Input: part model. Units: mm. Frame: model coordinates. A direction names the side the tool comes from. Round coordinates to 2 decimals unless told otherwise and drop trailing zeros. Order: outer loops, then holes, each group sorted by start corner. A loop starts at its lowest first (then second) coordinate and runs counter-clockwise, first axis right, second up. Notation, with made-up numbers: (38.5, 56) - (58.5, 56) arc R23 cw to (58.5, 93) - close; hole circle Ø2 at (1.5, 87.5). An arc over 180 degrees is marked (long way). One line per item, written item: value. Start each with the question number.
from build123d import *

# Parameters (mm, degrees)
F0_W     = 132.842
F0_H     = 119.38
F1_DEPTH = 88.392
F2_R     = 40.132
F3_DEPTH = 120.396
F4_R     = 9.525
F5_DEPTH = 79.502


with BuildPart() as f1:
    # F0 (on Front) → F1 (new body)
    with BuildSketch(Plane.XZ):
        with Locations((-0.909254, 5.516134)):
            Rectangle(F0_W, F0_H)
    extrude(amount=-F1_DEPTH)

    # F2 (on face) → F3 (join)
    with BuildSketch(Plane.XY.offset(65.206134)):
        with Locations((40.111746, 37.592)):
            Circle(F2_R)
    extrude(amount=F3_DEPTH)

    # F4 (on face) → F5 (join)
    with BuildSketch(Plane.XZ):
        with Locations((-12.720254, 1.706134)):
            Circle(F4_R)
    extrude(amount=F5_DEPTH)


solid = f1.part
1. Pin query (flat end, axial travel): pin 1 (1.5 mm diameter, centred on y = 70, z = 31, fed in from +X); pin 2 (6 mm diameter, centred on x = 15, z = 134, fed in from -Y); pin 3 (3 mm diameter, centred on x = 38, z = 66.5, fed in from -Y). Return the tip coordinate at first contact, or that it passes through.
2. Section B-B (x = -32.5). Return the cut outline in (y, z).
3. Section D-D (z = 134). Return the cut outline in (x, y).
4. Line query: line 1 (Y direction, x = -20, z = -43.5); line 2 (Z direction, x = -13.5, y = 39); line 3 (X direction, y = 61, z = -3.5). Output: solid intervals per line, ascending. Write a range as from..to.
5. Section C-C (y = -52). Return the cut outline in (x, z) (3 decimals).
6. Set-up query: faces 1 (the face through (62, 2, 65.206)), 2 (the face through (65.512, 44, 5)), 3 (the face through (-3.635, -39.194, 4.567)). Return all of +Z, -Z, +X, -X, +Y, -Y with unobstructed straight access to the full face (end or side cutting, diameter ignored); none if empty.
7. Section A-A (z = 62.5). Return the cut outline in (x, y).
Solved:
1. pin 1: stops at x = 65.51
1. pin 2: stops at y = 4.1
1. pin 3: stops at y = -2.54
2. outline: (0, -54.17) - (88.39, -54.17) - (88.39, 65.21) - (0, 65.21) - close
3. outline: circle Ø80.26 at (40.11, 37.59)
4. line 1: y = 0..88.39
4. line 2: z = -54.17..65.21
4. line 3: x = -67.33..65.51
5. outline: circle Ø19.05 at (-12.72, 1.706)
6. face 1: +Z, +X, -Y
6. face 2: -Z, +X, +Y, -Y
6. face 3: -Y
7. outline: (-67.33, 0) - (65.51, 0) - (65.51, 88.39) - (-67.33, 88.39) - close
